Source: CAD feature listing. Evaluate the final solid. Frame: model axes, mm. Give positions to 0.01 mm unless a question says otherwise; leave off trailing zeros. Order: outer loops, then holes, each group sorted by start corner. A loop starts at its lowest first (then second) coordinate and runs counter-clockwise, first axis right, second up.
from build123d import *

# Parameters (mm, degrees)
SKETCH1_R               = 19.05
SKETCH1_R_2             = 8.001
BOSS_EXTRUDE1_DEPTH     = 3.175
SKETCH2_R               = 19.05
BOSS_EXTRUDE2_DEPTH     = 4.7625
F_3_8_CLEARANCE_HOLE1_D = 10.31748
SKETCH6_R               = 8.001
CUT_EXTRUDE1_DEPTH      = 2.54
SKETCH7_R               = 19.05
CUT_EXTRUDE2_DEPTH      = 2.2225
SKETCH8_R               = 28.575
SKETCH8_R_2             = 19.05
BOSS_EXTRUDE3_DEPTH     = 5.715


with BuildPart() as part:
    # Sketch1 → Boss-Extrude1 (new body)
    with BuildSketch(Plane.XY):
        with Locations((95.864074702, 45.465579041)):
            Circle(SKETCH1_R)
        with Locations((95.864074702, 45.465579041)):
            Circle(SKETCH1_R_2, mode=Mode.SUBTRACT)
    extrude(amount=-BOSS_EXTRUDE1_DEPTH)

    # Sketch2 → Boss-Extrude2 (add)
    with BuildSketch(Plane.XY):
        with Locations((95.864074702, 45.465579041)):
            Circle(SKETCH2_R)
    extrude(amount=BOSS_EXTRUDE2_DEPTH)

    # 3/8 Clearance Hole1 (through all)
    with Locations(Plane.XY.offset(4.7625)):
        with Locations((95.864074702, 45.465579041)):
            Hole(F_3_8_CLEARANCE_HOLE1_D / 2)

    # Sketch6 → Cut-Extrude1 (cut)
    with BuildSketch(Plane(origin=(0, 0, 0), x_dir=(-1, 0, 0), z_dir=(0, 0, -1))):
        with Locations((-95.864074702, 45.465579041)):
            Circle(SKETCH6_R)
    extrude(amount=-CUT_EXTRUDE1_DEPTH, mode=Mode.SUBTRACT)

    # Sketch7 → Cut-Extrude2 (cut)
    with BuildSketch(Plane.XY.offset(4.7625)):
        with Locations((95.864074702, 45.465579041)):
            Circle(SKETCH7_R)
    extrude(amount=-CUT_EXTRUDE2_DEPTH, mode=Mode.SUBTRACT)

    # Sketch8 → Boss-Extrude3 (add)
    with BuildSketch(Plane(origin=(0, 0, -3.175), x_dir=(-1, 0, 0), z_dir=(0, 0, -1))):
        with Locations((-95.864074702, 45.465579041)):
            Circle(SKETCH8_R)
        with Locations((-95.864074702, 45.465579041)):
            Circle(SKETCH8_R_2, mode=Mode.SUBTRACT)
    extrude(amount=-BOSS_EXTRUDE3_DEPTH)


solid = part.part
1) Section query B-B on x = 93.5. Output: boundary loops of the cut face in (y, z) (3 decimals).
Checks:
outline: (16.989, -3.175) - (37.822, -3.175) - (37.822, 2.54) - (16.989, 2.54) - close; (53.109, -3.175) - (73.943, -3.175) - (73.943, 2.54) - (53.109, 2.54) - close
2) Section query C-C on z = -1.15. Output: boundary loops of the cut face in (x, y) (3 decimals), and give its area (3 significant figures).
Checks:
outline: circle Ø57.15 at (95.864, 45.466); hole circle Ø16.002 at (95.864, 45.466)
area: 2,360 mm2
3) Section query A-A on y = 39. Output: boundary loops of the cut face in (x, z) (3 decimals).
Checks:
outline: (68.03, -3.175) - (91.151, -3.175) - (91.151, 2.54) - (68.03, 2.54) - close; (100.577, -3.175) - (123.698, -3.175) - (123.698, 2.54) - (100.577, 2.54) - close
4) Section query D-D on x = 81.5. Output: boundary loops of the cut face in (y, z) (3 decimals).
Checks:
outline: (20.763, -3.175) - (70.168, -3.175) - (70.168, 2.54) - (20.763, 2.54) - close
5) Ray query, L1, parallel to X at y = 50, z = -2; L2, parallel to X at y = 46.5, z = 1.9; L3, parallel to Y at x = 117.5, z = 1.05. Return the intervals inside material, ascending.
Checks:
L1: x = 67.65 to 89.27, 102.46 to 124.08
L2: x = 67.31 to 87.93, 103.8 to 124.42
L3: y = 26.8 to 64.13
6) First-contact query: pin 1 Ø9.5 at (x, y) = (95.86, 45.47) entering from +Z; pin 2 Ø1.5 at (x, z) = (84, 1.5) entering from -Y; pin 3 Ø2 at (y, z) = (56.5, -2) entering from -X; pin 4 Ø2 at (y, z) = (31.5, 0) entering from +X. Flat tips, straight axial feed; report the tip coordinate or a pass-through.
Checks:
pin 1: passes through
pin 2: stops at y = 19.14
pin 3: stops at x = 69.11
pin 4: stops at x = 121.33
